```python
from build123d import *

# Parameters (mm, degrees)
SKETCH1_W               = 100
SKETCH1_H               = 60
BOSS_EXTRUDE1_DEPTH     = 40
BOSS_EXTRUDE2_DEPTH     = 85
CUT_EXTRUDE1_DEPTH      = 110.36175698
CUT_EXTRUDE1_DEPTH_BACK = 110.36175698
SKETCH3_R               = 4.7625
SKETCH5_W               = 20
SKETCH5_H               = 25.4
BOSS_EXTRUDE3_DEPTH     = 40
CUT_EXTRUDE2_DEPTH      = 110.36175698
CUT_EXTRUDE2_DEPTH_BACK = 110.36175698
SKETCH4_R               = 4.7625
CUT_EXTRUDE3_START      = -40
SKETCH6_R               = 4.7625
CUT_EXTRUDE3_DEPTH      = 40


with BuildPart() as part:
    # Sketch1 → Boss-Extrude1 (new, symmetric)
    with BuildSketch(Plane(origin=(0, 0, 0), x_dir=(1, 0, 0), z_dir=(0, 1, 0))):
        Rectangle(SKETCH1_W, SKETCH1_H)
    extrude(amount=BOSS_EXTRUDE1_DEPTH, both=True)

    # Sketch2 → Boss-Extrude2 (add)
    with BuildSketch(Plane.XY.offset(30)):
        Polygon((43.291016151, 10.998522628), (30.300635095, 3.498522628), (43.000635095, -18.498522628), (55.991016151, -10.998522628), align=None)
    extrude(amount=BOSS_EXTRUDE2_DEPTH)

    # Sketch3 → Cut-Extrude1 (cut, two sides: drawn at the far end of the back side and taken through both)
    with BuildSketch(Plane.XY.offset(30).offset(-CUT_EXTRUDE1_DEPTH_BACK)):
        with Locations((15, -20)):
            Circle(SKETCH3_R)
    extrude(amount=CUT_EXTRUDE1_DEPTH + CUT_EXTRUDE1_DEPTH_BACK, mode=Mode.SUBTRACT)

    # Sketch5 → Boss-Extrude3 (add)
    with BuildSketch(Plane(origin=(24.240381057, 13.995190528, 0), x_dir=(0, 0, 1), z_dir=(-0.866025403784436, -0.5000000000000046, 0))):
        with Locations((105, -24.820508076)):
            Rectangle(SKETCH5_W, SKETCH5_H)
    extrude(amount=BOSS_EXTRUDE3_DEPTH)

    # Sketch4 → Cut-Extrude2 (cut, two sides: drawn at the far end of the back side and taken through both)
    with BuildSketch(Plane.XY.offset(30).offset(-CUT_EXTRUDE2_DEPTH_BACK)):
        with Locations((-5, 5)):
            Circle(SKETCH4_R)
    extrude(amount=CUT_EXTRUDE2_DEPTH + CUT_EXTRUDE2_DEPTH_BACK, mode=Mode.SUBTRACT)

    # Sketch6 → Cut-Extrude3 (cut)
    with BuildSketch(Plane(origin=(0, 0, 95), x_dir=(-1, 0, 0), z_dir=(0, 0, -1)).offset(CUT_EXTRUDE3_START)):
        with Locations(Location((-15, -20, 0), (0, 0, 180))):
            Circle(SKETCH6_R)
    extrude(amount=CUT_EXTRUDE3_DEPTH, mode=Mode.SUBTRACT)


solid = part.part
```
Part model, mm, in its own coordinate system. A direction names the side the tool comes from. Round coordinates to 2 decimals unless told otherwise and drop trailing zeros. Write each loop counter-clockwise with the first axis right and the second up, starting at its lowest first coordinate (ties: lowest second). Pieces come first, ordered by that corner, then holes. Notation, with made-up numbers: (35, 28) -> (70, 28) arc R13 cw to (70, 46) -> close; hole circle Ø4 at (86, 12.5). An arc over 180 degrees is marked (long way). Return JSON: item names as keys, results as strings. Group by question number.
Q1. Probe L1, parallel to Y at x = -5.5, z = 10; L2, parallel to Y at x = -5, z = 10; L3, parallel to Z at x = -33.5, y = 1.5. List the from-to ranges inside material, lowest first. Write a range as [from, to].
Q2. Saw through at D-D on x = -34. Write the cut outline in (y, z).
Q3. Saw through at B-B on z = -9. Write the cut outline in (x, y) (1 decimal).
Q4. Mould opens along Y. For faces 6 (the cylindrical face through (13.97, -15.35, 105.14)), 7 (the flat face through (36.562, -7.346, 62.045)), 8 (the flat face through (52, -9, 30)) say: pulls with the +Y half, pulls with the -Y half, needs draft (parallel to the pull), parting line crosses it, or undercut.
Q5. Pin check, flat tips, straight feed: pin 1 (5 mm diameter, centred on x = 54.5, y = -10.5, fed in from -Z); pin 2 (12 mm diameter, centred on y = -1, z = 65.5, fed in from +X); pin 3 (12.5 mm diameter, centred on x = 15, y = -20, fed in from -Z); pin 4 (10 mm diameter, centred on x = 39.5, y = 17.5, fed in from +Z). Stop position of each tip, or through.
Q6. Saw through at C-C on z = 69.5. Write the cut outline in (x, y), plus the area to 3 significant figures.
Q7. Which spindle directions (+Z, -Z, +X, -X, +Y, -Y) get a long thin tool onto all of the face, cutting with end or side? Do faces 1 (the flat face through (49.73, -0.154, 71.905)), 2 (the flat face through (-50, 1, 0)), 3 (the cylindrical face through (13.97, -24.65, -0.42)), 4 (the flat face through (1.921, -27.346, 104.86)), 5 (the flat face through (20, -18, 95)). Say none if no direction does.
Q8. Saw through at A-A on x = 15. Write the cut outline in (y, z), plus the area to 3 significant figures.
Answer:
{
 "1": {"L1": "[-40, 0.26], [9.74, 40]", "L2": "[-40, 0.24], [9.76, 40]", "L3": "[-30, 30]"},
 "2": {"outline": "(-40, -30) -> (40, -30) -> (40, 30) -> (-40, 30) -> close"},
 "3": {"outline": "(-50, -40) -> (50, -40) -> (50, 40) -> (-50, 40) -> close; hole circle Ø9.5 at (-5, 5); hole circle Ø9.5 at (15, -20)"},
 "4": {"face 6": "undercut", "face 7": "pulls with the -Y half", "face 8": "needs draft"},
 "5": {"pin 1": "z = 30", "pin 2": "x = 53.68", "pin 3": "z = -30", "pin 4": "z = 30"},
 "6": {"outline": "(30.3, 3.5) -> (43, -18.5) -> (55.99, -11) -> (43.29, 11) -> close", "area": "381 mm2"},
 "7": {"face 1": "+Z, +X, +Y", "face 2": "+Z, -Z, -X, +Y, -Y", "face 3": "+Z, -Z", "face 4": "+Z, -X, -Y", "face 5": "-X, -Y"},
 "8": {"outline": "(-40, -30) -> (-24.76, -30) -> (-24.76, 30) -> (-40, 30) -> close; (-34.66, 95) -> (-24.76, 95) -> (-24.76, 115) -> (-34.66, 115) -> close; (-15.24, -30) -> (40, -30) -> (40, 30) -> (-15.24, 30) -> close; (-15.24, 95) -> (-5.34, 95) -> (-5.34, 115) -> (-15.24, 115) -> close", "area": "4,620 mm2"}
}
